Check sheet for the modelled part. Datum: model origin and axes. Units: mm. Face numbers are marked on the shaded views. Coordinates: 2 decimals unless noted, no trailing zeros. Loops run counter-clockwise (first coordinate to the right, second up) from the corner with the lowest first, then second, coordinate; pieces in that order, holes last. Notation, with made-up numbers: M 44,-39.75 L 51,-39.75 A20 cw 51,-32.75 Z; hole C -30,-12.75 d8. An arc over 180 degrees is marked long. Write each question's results on one line, items separated by ' | '. Start each with the question number.
Autodesk Inventor part; units mm, degrees
ref_plane "YZ Plane" through (0, 0, 0) normal (1, 0, 0) x (0, 1, 0)
ref_plane "XZ Plane" through (0, 0, 0) normal (0, 1, 0) x (-1, 0, 0)
ref_plane "XY Plane" through (0, 0, 0) normal (0, 0, 1) x (1, 0, 0)
sketch "Sketch2" plane through (0, 0, 0) normal (0, 0, 1) x (1, 0, 0)
  line L0 (-14.9328, -5.3201) -> (-10.9328, -5.3201)
  line L1 (-10.9328, -5.3201) -> (-10.9328, -11.3201)
  line L2 (20.0672, -9.3201) -> (20.0672, -9.3157)
  line L3 (-6.9328, -9.3201) -> (-6.9328, -1.3201)
  line L4 (-6.9328, -1.3201) -> (-14.9328, -1.3201)
  line L5 (-14.9328, -1.3201) -> (-14.9328, -5.3201)
  line L6 (-14.9328, -5.3201) -> (-10.9328, -5.3201)
  line L7 (-14.9328, -1.3201) -> (-6.9328, -1.3201)
  line L8 (-6.9328, -1.3201) -> (-6.9328, -9.3201)
  line L9 (16.0672, -9.3157) -> (16.0672, -9.3201)
  line L10 (-10.9328, -11.3201) -> (-10.9328, -5.3201)
  line L11 (-10.9328, -5.3201) -> (-14.9328, -5.3201)
  line L12 (-14.9328, -1.3201) -> (-14.9328, -5.3201)
  line L13 (-10.9328, -11.3201) -> (34.4422, -11.3201)
  line L14 (-10.9328, -11.3201) -> (34.4422, -11.3201) construction
  line L15 (34.4422, -11.3201) -> (34.4422, -9.3201)
  line L16 (-6.9328, -9.3201) -> (34.4422, -9.3201)
  point P0 (0, 0)
  point P1 (-14.9328, 16.2146)
  point P2 (20.0672, -10.3179)
  point P3 (-12.9328, -5.3201)
  point P4 (-14.9328, -5.3201)
  dimension "d2" = 8
  dimension "d3" = 90
  dimension "d4" = 4
  dimension "d5" = 90
  dimension "d6" = 4
  dimension "d7" = 90
  dimension "d23" = 45.375
  dimension "d24" = 0
  dimension "d25" = 2
extrude "Extrusion4" add sketch "Sketch2" along normal blind 83.525
mirror "Mirror4" about plane through (34.4422, -11.3201, 0) normal (1, 0, 0) of "Extrusion4"
properties part number "Avionics Cradle (12-13)"
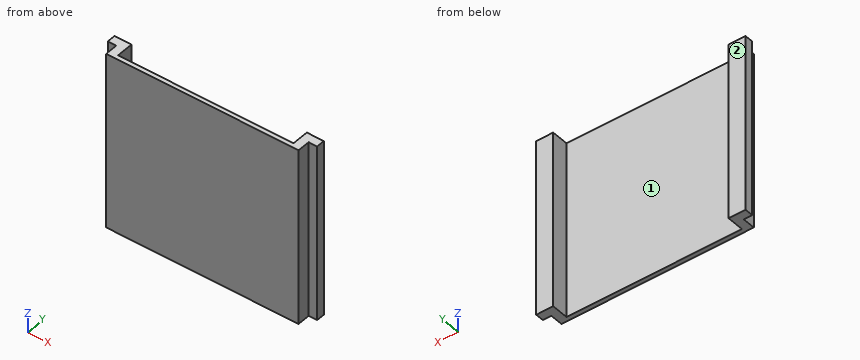
1) Thickness scan on probe 1 along X at (y, z) = (-3.25, 39.5); probe 2 along X at (y, z) = (-8.5, 25); probe 3 along Y at (x, z) = (13, 71.5). Record the ranges inside material, lowest first.
2) Section check C-C (x = 46). Enter the section's corners in (y, z) (3 decimals).
3) Section check B-B (z = 36.5). Enter the section's corners in (x, y).
4) Gauge pin test, flat ends, axial feed: P1, Ø4, axis at x = 35.5, z = 62, coming from the +Y side; P2, Ø3, axis at x = 82, z = 46, coming from the -Y side. Record the tip position at first contact, or that the pin passes through.
5) Release check for a two-part mould opening along X. For the marked faces 1 and 2 record: +X half, -X half, draft (parallel to the pull), parting line (faces both ways), or undercut.
6) Section check A-A (y = -3.25). Enter the section's corners in (x, z) (3 decimals), then the cut area to 3 significant figures.
Return value:
1) probe 1: x = -14.93 to -6.93, 75.82 to 83.82 | probe 2: x = -10.93 to -6.93, 75.82 to 79.82 | probe 3: y = -11.32 to -9.32
2) outline: M -11.32,0 L -9.32,0 L -9.32,83.525 L -11.32,83.525 Z
3) outline: M -14.93,-5.32 L -10.93,-5.32 L -10.93,-11.32 L 79.82,-11.32 L 79.82,-5.32 L 83.82,-5.32 L 83.82,-1.32 L 75.82,-1.32 L 75.82,-9.32 L -6.93,-9.32 L -6.93,-1.32 L -14.93,-1.32 Z
4) P1: stops at y = -9.32 | P2: stops at y = -5.32
5) face 1: undercut | face 2: draft
6) outline: M -14.933,0 L -6.933,0 L -6.933,83.525 L -14.933,83.525 Z; M 75.817,0 L 83.817,0 L 83.817,83.525 L 75.817,83.525 Z | area: 1,340 mm2
